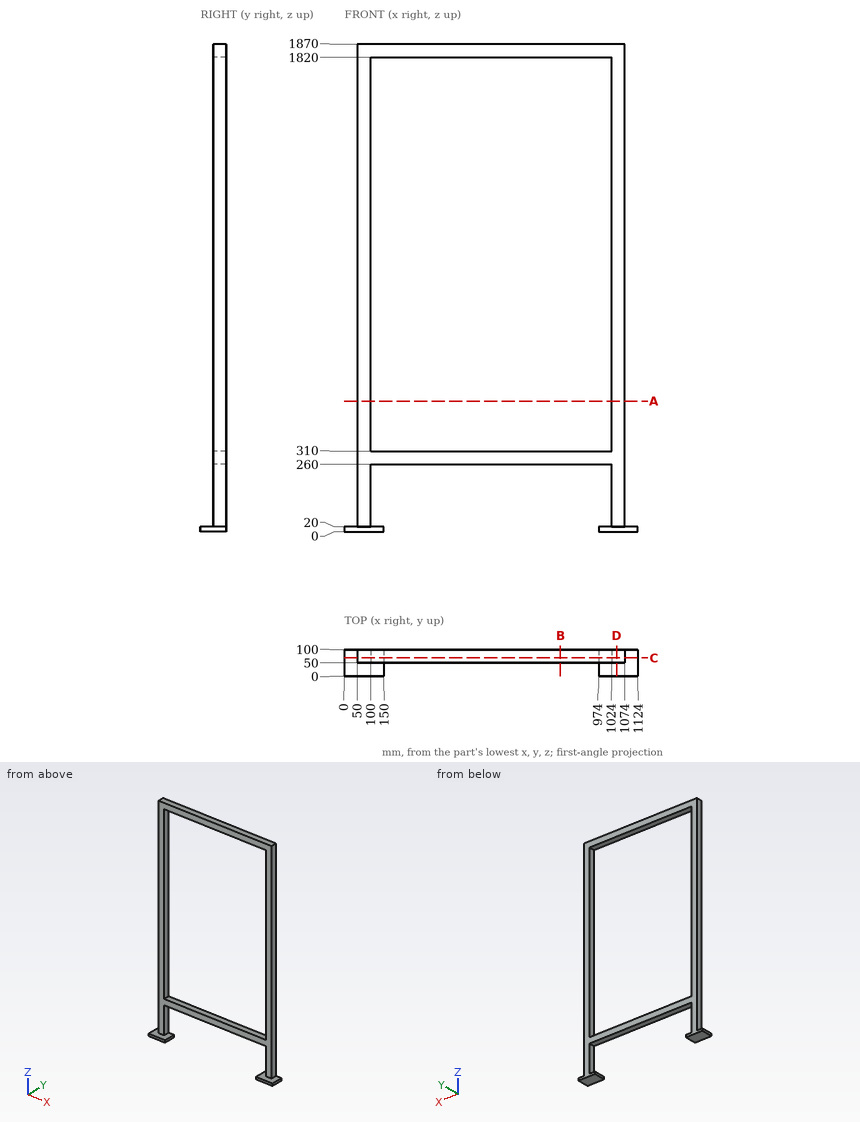
Geometry: see drawing. Coordinates: mm, zero at the bounding-box minimum. Give positions to 0.01 mm unless a question says otherwise; leave off trailing zeros. Loops run counter-clockwise (first coordinate to the right, second up) from the corner with the lowest first, then second, coordinate; pieces in that order, holes last. Notation, with made-up numbers: (-21.75, -7) - (-9.75, -7) arc R5 ccw to (-9.75, -1) - close; hole circle Ø10 at (-3, -33.75). An arc over 180 degrees is marked (long way). One line per question, with ' | ' between items. Start each with the question number.
(1) Section query A-A on z = 501. Return loops of the section in (x, y), then the cut area to 3 significant figures.
(2) Section query D-D on x = 1043.5. Return loops of the section in (y, z).
(3) Ray query, line 1 (X direction, y = 78, z = 1648.5); line 2 (Z direction, x = 552, y = 66.5); line 3 (Z direction, x = 988, y = 55.5). Return the intervals inside material, ascending. Write a range as from..to.
(4) Contact query for flat-ended pins moving along their axis: pin 1 (25 mm diameter, centred on y = 71, z = 991, fed in from +X); pin 2 (4 mm diameter, centred on y = 72.5, z = 1154.5, fed in from -X); pin 3 (10 mm diameter, centred on x = 258, y = 70.5, fed in from -Z). Output: stop coordinate, or through.
(5) Section query C-C on y = 69. Return loops of the section in (x, z).
(6) Section query B-B on x = 828. Return loops of the section in (y, z), then the cut area to 3 significant figures.
The answers:
1) outline: (50, 50) - (100, 50) - (100, 100) - (50, 100) - close; (1024, 50) - (1074, 50) - (1074, 100) - (1024, 100) - close | area: 5,000 mm2
2) outline: (0, 0) - (100, 0) - (100, 1870) - (50, 1870) - (50, 20) - (0, 20) - close
3) line 1: 50..100, 1024..1074 | line 2: 260..310, 1820..1870 | line 3: 0..20, 260..310, 1820..1870
4) pin 1: x = 1074 | pin 2: x = 50 | pin 3: z = 260
5) outline: (0, 0) - (150, 0) - (150, 20) - (100, 20) - (100, 260) - (1024, 260) - (1024, 20) - (974, 20) - (974, 0) - (1124, 0) - (1124, 20) - (1074, 20) - (1074, 1870) - (50, 1870) - (50, 20) - (0, 20) - close; hole (100, 310) - (1024, 310) - (1024, 1820) - (100, 1820) - close
6) outline: (50, 260) - (100, 260) - (100, 310) - (50, 310) - close; (50, 1820) - (100, 1820) - (100, 1870) - (50, 1870) - close | area: 5,000 mm2
